```python
from build123d import *

# Parameters (mm, degrees)
F0_W     = 127
F0_H     = 127
F1_DEPTH = 12.7
F2_W     = 12.7
F2_H     = 12.7
F2_R     = 6.35
F3_DEPTH = 76.2


# Not quite as in the source:
# - a feature names something its author has since deleted; it is built from what else it names


with BuildPart() as f1:
    # F0 (on Top) → F1 (new body)
    with BuildSketch(Plane.XY):
        with Locations((-63.5, -63.5)):
            Rectangle(F0_W, F0_H)
    extrude(amount=F1_DEPTH)

    # F2 (on face) → F3 (join)
    with BuildSketch(Plane.XY.offset(12.7)):
        with Locations((-120.65, -6.35)):
            Rectangle(F2_W, F2_H)
        with Locations((-6.35, -6.35)):
            Rectangle(F2_W, F2_H)
        with Locations((-120.1874390244, -120.5023750663)):
            Circle(F2_R)
        with Locations((-6.6746613011, -120.3140169382)):
            Circle(F2_R)
    extrude(amount=F3_DEPTH)


solid = f1.part
```
Part model, mm, in its own coordinate system. A direction names the side the tool comes from. Round coordinates to 2 decimals unless told otherwise and drop trailing zeros. Loops run counter-clockwise (first coordinate to the right, second up) from the corner with the lowest first, then second, coordinate; pieces in that order, holes last.
Item 1: Drop flat-ended pins along their axis: P1, Ø10, axis at x = -15.5, z = 56.5, coming from the -Y side; P2, Ø6, axis at x = -35.5, z = 17.5, coming from the +Y side; P3, Ø14, axis at x = -118, z = 49, coming from the -Y side; P4, Ø6.5, axis at x = -4, z = 45.5, coming from the -Y side. Give the stop position or say it passes through.
Item 2: Cut at B-B, the plane x = -116. Give the cut face in (y, z).
Item 3: Mould opens along Y. For faces 1 (the face through (-114.3, -6, 50)), 2 (the face through (-64, -127, 6)), 3 (the face through (-7.501, -114.018, 50.267)) say: +Y half, -Y half, draft (parallel to the pull), parting line (faces both ways), or undercut.
Item 4: Cut at C-C, the plane y = -73.5. Give the cut face in (x, z), then the cut area to 3 significant figures.
Item 5: 3-axis set-ups, long thin cutter, end or side, ignore diameter. For faces 4 (the face through (-12.7, -6, 50)), 5 (the face through (-116.77, -115.15, 50.27)), 6 (the face through (-6, -12.7, 50)), 7 (the face through (-7, -120, 88.9)): which of +Z, -Z, +X, -X, +Y, -Y reach the whole face in a straight line?
Item 6: Drill centre lines: line 1 (X direction, y = -10.5, z = 38); line 2 (Z direction, x = -90.5, y = -77.5); line 3 (X direction, y = -117, z = 70.5). Where is each one in solid material? Low to high.
Item 7: Cut at A-A, the plane z = 15. Give the cut face in (x, y), then the cut area to 3 significant figures.
A:
1. P1: stops at y = -125.38
1. P2: passes through
1. P3: stops at y = -126.85
1. P4: stops at y = -126.66
2. outline: (-127, 0) - (0, 0) - (0, 88.9) - (-12.7, 88.9) - (-12.7, 12.7) - (-115.73, 12.7) - (-115.73, 88.9) - (-125.28, 88.9) - (-125.28, 12.7) - (-127, 12.7) - close
3. face 1: draft
3. face 2: -Y half
3. face 3: undercut
4. outline: (-127, 0) - (0, 0) - (0, 12.7) - (-127, 12.7) - close
4. area: 1,610 mm2
5. face 4: +Z, +Y
5. face 5: +Z
5. face 6: +Z, +X, -X
5. face 7: +Z, +X, -X, +Y, -Y
6. line 1: x = -127 to -114.3, -12.7 to 0
6. line 2: z = 0 to 12.7
6. line 3: x = -125.48 to -114.89, -12.09 to -1.26
7. outline: (-127, -12.7) - (-114.3, -12.7) - (-114.3, 0) - (-127, 0) - close; circle Ø12.7 at (-120.19, -120.5); circle Ø12.7 at (-6.67, -120.31); (-12.7, -12.7) - (0, -12.7) - (0, 0) - (-12.7, 0) - close
7. area: 576 mm2
